Study the drawing (mm; zero at the part's minimum x, y, z) and answer. A direction names the side the tool comes from. Give positions to 0.01 mm unless a question says otherwise; leave off trailing zeros. Write each loop counter-clockwise with the first axis right and the second up, starting at its lowest first coordinate (ties: lowest second). Pieces come first, ordered by that corner, then holes. Notation, with made-up numbers: (44, 30) - (64, 30) arc R18 ccw to (64, 60) - close; hole circle Ø10 at (54, 80). An arc over 180 degrees is marked (long way). One line per item, written item: value. Start each with the question number.
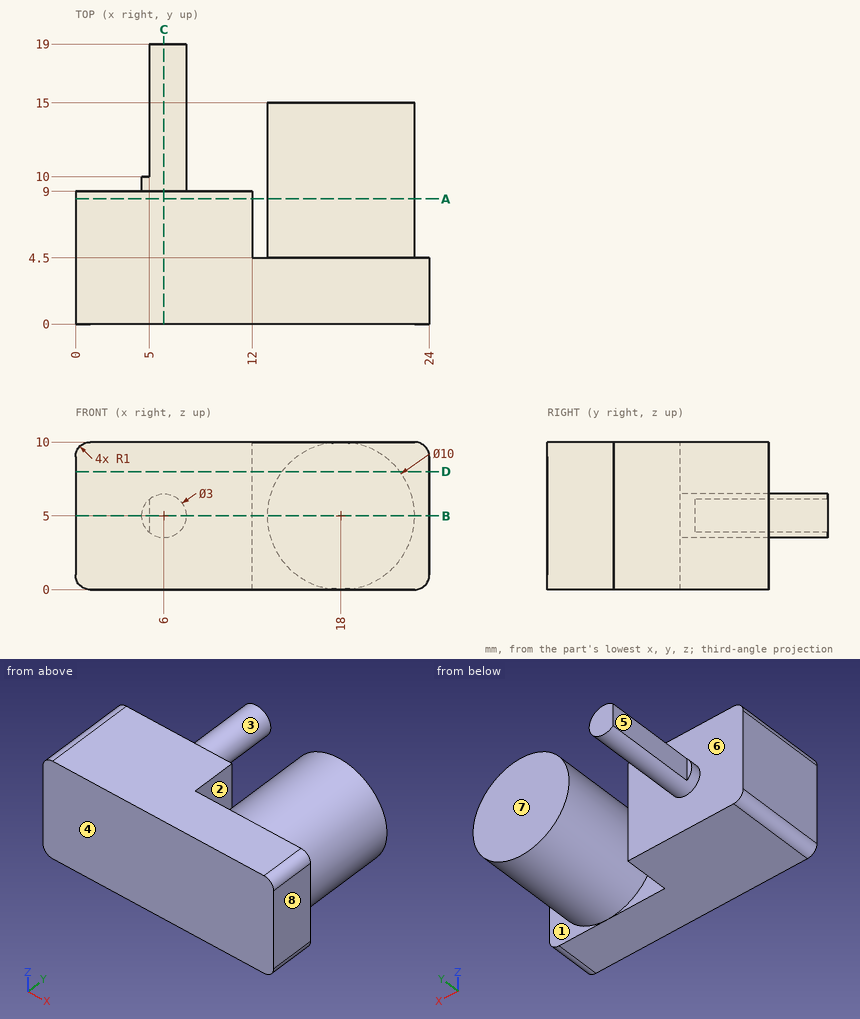
Item 1: Each of these flat-tipped pins is pushed along its axis until it touches: pin 1 Ø1.8 at (y, z) = (15.5, 5.5) entering from -X; pin 2 Ø1.5 at (y, z) = (13, 4.5) entering from +X; pin 3 Ø3 at (x, z) = (14.5, 4.5) entering from +Y. Where does it stop, or does it pass through?
Item 2: Find section D-D on z = 8. Determine the outline of the cut face in (x, y).
Item 3: Straight lines are drawn through the part: line 1 along Y through (x, z) = (8.75, 8); line 2 along Y through (x, z) = (17.75, 7); line 3 along X through (y, z) = (8.5, 8). For each, find the intervals that lie inside material, in ascending order.
Item 4: Find section B-B on z = 5. Determine the outline of the cut face in (x, y), plus the area to 4 significant figures.
Item 5: The mould has two halves that part along X. Classify the marked faces 6, 7 and 8: +X half, -X half, draft (parallel to the pull), parting line (faces both ways), or undercut.
Item 6: For the marked faces 1, 2, 3, 4 and 5, determine the directions among +Z, -Z, +X, -X, +Y, -Y from which every point of the face is accessible in a straight line to the end or side of a thin tool.
Item 7: Find section A-A on y = 8.5. Determine the outline of the cut face in (x, z), plus the area to 3 significant figures.
Item 8: Find section C-C on x = 6. Determine the outline of the cut face in (y, z).
Values:
1. pin 1: x = 5
1. pin 2: x = 23
1. pin 3: y = 15
2. outline: (0, 0) - (24, 0) - (24, 4.5) - (22, 4.5) - (22, 15) - (14, 15) - (14, 4.5) - (12, 4.5) - (12, 9) - (0, 9) - close
3. line 1: 0 to 9
3. line 2: 0 to 15
3. line 3: 0 to 12, 14 to 22
4. outline: (0, 0) - (24, 0) - (24, 4.5) - (23, 4.5) - (23, 15) - (13, 15) - (13, 4.5) - (12, 4.5) - (12, 9) - (7.5, 9) - (7.5, 19) - (5, 19) - (5, 10) - (4.5, 10) - (4.5, 9) - (0, 9) - close
4. area: 292.5 mm^2
5. face 6: undercut
5. face 7: draft
5. face 8: +X half
6. face 1: +X, +Y
6. face 2: +Z, -Z, +Y
6. face 3: +Y
6. face 4: +Z, -Z, +X, -X, -Y
6. face 5: +Z, -Z, -X, +Y
7. outline: (0, 1) arc R1 ccw to (1, 0) - (12, 0) - (12, 10) - (1, 10) arc R1 ccw to (0, 9) - close; circle Ø10 at (18, 5)
7. area: 198 mm^2
8. outline: (0, 0) - (9, 0) - (9, 3.5) - (19, 3.5) - (19, 6.5) - (9, 6.5) - (9, 10) - (0, 10) - close
